Study the drawing (mm; zero at the part's minimum x, y, z) and answer. Coordinates: 2 decimals unless noted, no trailing zeros. Loops run counter-clockwise (first coordinate to the right, second up) from the corner with the lowest first, then second, coordinate; pieces in that order, holes last. Notation, with made-up numbers: (-36, 56) -> (23, 56) arc R25 cw to (23, 83) -> close; hole circle Ø7 at (-21.5, 64.5). An arc over 180 degrees is marked (long way). Answer in a Markdown table with one row per item.
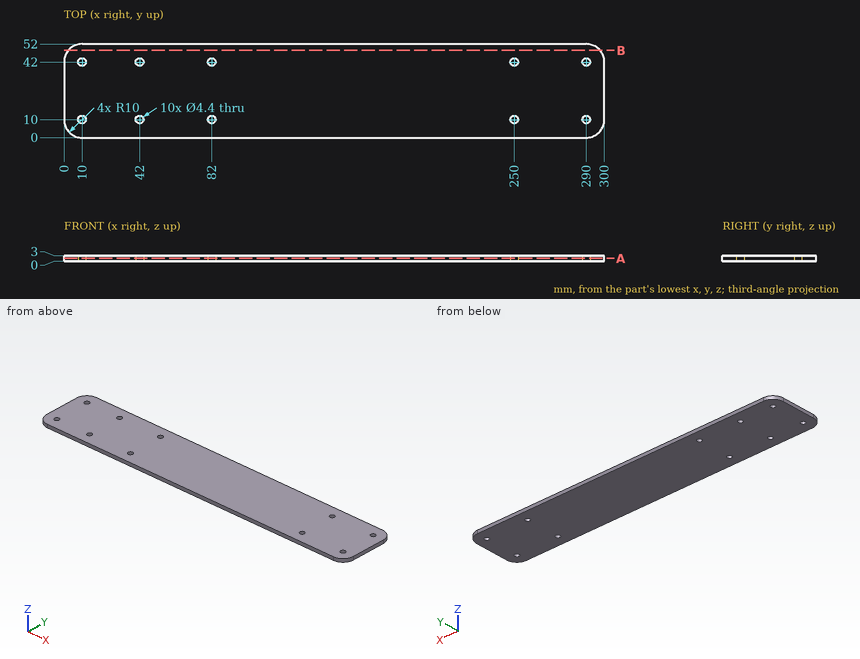
1. A cutting plane is placed at A-A on z = 1.55. Count the separate pieces of the cut face and the enclosed holes in it, and give its area (3 significant figures).
A:
| item | result |
|---|---|
| separate pieces | 1 |
| enclosed holes | 10 |
| area | 15,400 mm2 |
2. A cutting plane is placed at B-B on y = 48.5. Give the vertices of the cut face in (x, z).
A:
| item | result |
|---|---|
| outline | (2.4, 0) -> (297.6, 0) -> (297.6, 3) -> (2.4, 3) -> close |
3. Find the intervals of material crossed by probe 1 along Y at (x, z) = (290, 2.05); probe 2 along X at (y, z) = (40, 0.7); probe 3 along Y at (x, z) = (80.5, 2.85), in increasing order.
A:
| item | result |
|---|---|
| probe 1 | y = 0 to 7.8, 12.2 to 39.8, 44.2 to 52 |
| probe 2 | x = 0 to 9.08, 10.92 to 41.08, 42.92 to 81.08, 82.92 to 249.08, 250.92 to 289.08, 290.92 to 300 |
| probe 3 | y = 0 to 8.39, 11.61 to 40.39, 43.61 to 52 |
